Model file for the job. Use its own axes, mm. A direction names the side the tool comes from. Coordinates: 2 decimals unless noted, no trailing zeros. Write each loop counter-clockwise with the first axis right and the second up, starting at its lowest first coordinate (ties: lowest second). Pieces come first, ordered by that corner, then holes. Notation, with made-up numbers: (-31, 3.25) - (-9, 3.25) arc R21 cw to (-9, 26.25) - close; hole circle Ø7 at (63, -23). An arc over 180 degrees is marked (long way). Put each result on its own line as item: value. Start each with the question number.
1. Drill centre lines: L1, parallel to Y at x = 0, z = 64.8; L2, parallel to Y at x = 0, z = 0.3; L3, parallel to Z at x = 0, y = -3. Where is each one in solid material? Low to high. Write a range as from..to.
2. Saw through at B-B, the plane x = -1.5. Write the cut outline in (y, z).
3. Pull direction X, two halves, no side cores. Call faces 4 (the face through (4, -4, 65)), 5 (the face through (-1.08, -4.88, 64.75)), 6 (the face through (-1.172, 8.923, 32.045)): released by +X, released by -X, zero draft, split by the parting line, or undercut.
4. Saw through at A-A, the plane y = -2.5. Write the cut outline in (x, z), plus the area to 3 significant figures.
5. Which spindle directions (+Z, -Z, +X, -X, +Y, -Y) get a long thin tool onto all of the face, cutting with end or side? Do faces 1 (the face through (6.466, -2.681, 0.246)), 2 (the face through (0, -7.3, 0)), 3 (the face through (0, 0, 64.5)). Say none if no direction does.
6. Drop flat-ended pins along their axis: P1, Ø1.5, axis at y = -7, z = 20, coming from the -X side; P2, Ø4, axis at x = 4.5, z = 42.5, coming from the +Y side; P3, Ø9, axis at x = 0, y = 0, coming from the -Z side. Give the stop position or say it passes through.
7. Saw through at C-C, the plane z = 57. Write the cut outline in (x, y).
```python
from build123d import *

# Parameters (mm, degrees)
SKETCH1_R           = 9
BOSS_EXTRUDE1_DEPTH = 65
SKETCH2_R           = 7
CUT_EXTRUDE1_DEPTH  = 0.5
SKETCH3_R           = 5
CUT_EXTRUDE3_DEPTH  = 0.5


with BuildPart() as part:
    # Sketch1 → Boss-Extrude1 (new body)
    with BuildSketch(Plane.XY):
        Circle(SKETCH1_R)
    extrude(amount=BOSS_EXTRUDE1_DEPTH)

    # Sketch2 → Cut-Extrude1 (cut)
    with BuildSketch(Plane.XY):
        Circle(SKETCH2_R)
    extrude(amount=CUT_EXTRUDE1_DEPTH, mode=Mode.SUBTRACT)

    # Sketch3 → Cut-Extrude3 (cut)
    with BuildSketch(Plane.XY.offset(65)):
        Circle(SKETCH3_R)
    extrude(amount=-CUT_EXTRUDE3_DEPTH, mode=Mode.SUBTRACT)


solid = part.part
```
Final values:
1. L1: y = -9..-5, 5..9
1. L2: y = -9..-7, 7..9
1. L3: z = 0.5..64.5
2. outline: (-8.87, 0) - (-6.84, 0) - (-6.84, 0.5) - (6.84, 0.5) - (6.84, 0) - (8.87, 0) - (8.87, 65) - (4.77, 65) - (4.77, 64.5) - (-4.77, 64.5) - (-4.77, 65) - (-8.87, 65) - close
3. face 4: zero draft
3. face 5: undercut
3. face 6: split by the parting line
4. outline: (-8.65, 0) - (-6.54, 0) - (-6.54, 0.5) - (6.54, 0.5) - (6.54, 0) - (8.65, 0) - (8.65, 65) - (4.33, 65) - (4.33, 64.5) - (-4.33, 64.5) - (-4.33, 65) - (-8.65, 65) - close
4. area: 1,110 mm²
5. face 1: -Z
5. face 2: -Z, +X, -X, +Y, -Y
5. face 3: +Z
6. P1: stops at x = -6.48
6. P2: stops at y = 8.65
6. P3: stops at z = 0.5
7. outline: circle Ø18 at (0, 0)
